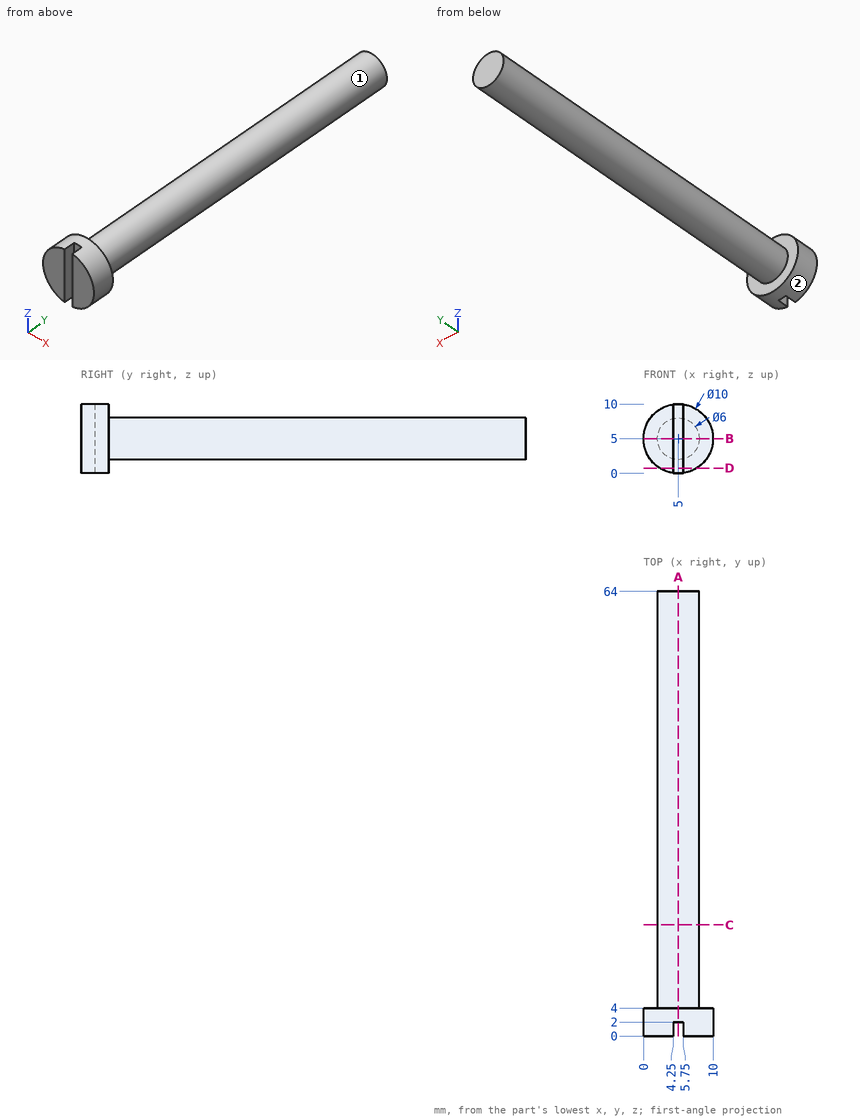
Geometry check sheet. Reference: drawing and pictorial views, mm from the part's lowest x, y, z. A direction names the side the tool comes from. Coordinates: 2 decimals unless noted, no trailing zeros. Order: outer loops, then holes, each group sorted by start corner. A loop starts at its lowest first (then second) coordinate and runs counter-clockwise, first axis right, second up. Notation, with made-up numbers: (-18, 20.5) - (35, 20.5) arc R6 cw to (35, 29.5) - close; hole circle Ø8 at (5, -5). An arc over 180 degrees is marked (long way). One line per item, written item: value.
(1) Depth check by flat-ended pin: pin 1 Ø1.5 at (x, y) = (4, 49.5) entering from +Z; pin 2 Ø1 at (y, z) = (1, 4) entering from +X; pin 3 Ø5 at (x, y) = (5, 26) entering from -Z. Enter the tip coordinate at first touch or a pass-through.
Data:
pin 1: stops at z = 7.99
pin 2: stops at x = 9.97
pin 3: stops at z = 2
(2) Sectioned sample at A-A (x = 5). Enter the section's corners in (y, z).
Data:
outline: (2, 0) - (4, 0) - (4, 2) - (64, 2) - (64, 8) - (4, 8) - (4, 10) - (2, 10) - close
(3) Sectioned sample at B-B (z = 5). Enter the section's corners in (x, y).
Data:
outline: (0, 0) - (4.25, 0) - (4.25, 2) - (5.75, 2) - (5.75, 0) - (10, 0) - (10, 4) - (8, 4) - (8, 64) - (2, 64) - (2, 4) - (0, 4) - close
(4) Access from +Z, -Z, +X, -X, +Y, -Y to the whole of each face (thin tool, end or side, straight path). Record for the marked faces 1 and 2.
Data:
face 1: +Y
face 2: +Y, -Y
(5) Sectioned sample at D-D (z = 0.75). Enter the section's corners in (x, y).
Data:
outline: (2.37, 0) - (4.25, 0) - (4.25, 2) - (5.75, 2) - (5.75, 0) - (7.63, 0) - (7.63, 4) - (2.37, 4) - close
(6) Sectioned sample at C-C (y = 16). Enter the section's corners in (x, z).
Data:
outline: circle Ø6 at (5, 5)
(7) Thickness scan on probe 1 along Y at (x, z) = (1, 4.5); probe 2 along X at (y, z) = (8, 3.75); probe 3 along Y at (x, z) = (4.5, 8.75). Record the ranges inside material, lowest first. Write a range as from..to.
Data:
probe 1: y = 0..4
probe 2: x = 2.27..7.73
probe 3: y = 2..4
